from build123d import *

# Parameters (mm, degrees)
EXTRUDE_START   = -375
EXTRUDE_1_DEPTH = 750


with BuildPart() as part:
    # Extrude sketch 1 → Extrude 1 (new body)
    with BuildSketch(Plane(origin=(0, 0, 0), x_dir=(1, 0, 0), z_dir=(0, 1, 0)).offset(EXTRUDE_START)):
        with BuildLine():
            Line((20, 16), (20, -16))
            ThreePointArc((20, -16), (18.828427125, -18.828427125), (16, -20))
            Line((16, -20), (-16, -20))
            ThreePointArc((-16, -20), (-18.828427125, -18.828427125), (-20, -16))
            Line((-20, -16), (-20, 16))
            ThreePointArc((-20, 16), (-18.828427125, 18.828427125), (-16, 20))
            Line((-16, 20), (16, 20))
            ThreePointArc((16, 20), (18.828427125, 18.828427125), (20, 16))
        make_face()
        with BuildLine():
            Line((17, 15.5), (17, -15.5))
            ThreePointArc((17, -15.5), (16.560660172, -16.560660172), (15.5, -17))
            Line((15.5, -17), (-15.5, -17))
            ThreePointArc((-15.5, -17), (-16.560660172, -16.560660172), (-17, -15.5))
            Line((-17, -15.5), (-17, 15.5))
            ThreePointArc((-17, 15.5), (-16.560660172, 16.560660172), (-15.5, 17))
            Line((-15.5, 17), (15.5, 17))
            ThreePointArc((15.5, 17), (16.560660172, 16.560660172), (17, 15.5))
        make_face(mode=Mode.SUBTRACT)
    extrude(amount=EXTRUDE_1_DEPTH)


solid = part.part
Here's how the part is built. I have some questions about the finished solid (model axes, mm). A direction names the side the tool comes from. Coordinates: 2 decimals unless noted, no trailing zeros. Loops run counter-clockwise (first coordinate to the right, second up) from the corner with the lowest first, then second, coordinate; pieces in that order, holes last. Notation, with made-up numbers: (-37.5, -28) -> (8.5, -28) arc R23 cw to (8.5, 9) -> close; hole circle Ø6 at (75, -18). An arc over 180 degrees is marked (long way). Use one line per item in the form item = value. Start each with the question number.
(1) If we section it at C-C (z = 9): Please give me the cut outline in (x, y).
(2) Will this pin go through, and if not, where does the flat tip stop? pin 1 (8 mm diameter, centred on x = 8.5, z = 9.5, fed in from -Y).
(3) We'd pull the mould along X, two halves only. Please class faces 1 (the face through (20, -5, 0)), 2 (the face through (18, -375, 0)), 3 (the face through (0, -5, 17)): pulls with the +X half, pulls with the -X half, needs draft (parallel to the pull), parting line crosses it, or undercut.
(4) On a 3-axis mill with a long thin cutter (end or side, diameter ignored), from which of +Z, -Z, +X, -X, +Y, -Y can I reach the whole of each face in a straight line? I mean faces 4 (the face through (0, -5, -17)), 5 (the face through (0, -5, -20)). Say none if no direction works.
(5) Please list where these lines run through material, in increasing order: line 1 along Z through (x, y) = (11, 138); line 2 along X through (y, z) = (-20.5, -16).
(6) If we section it at B-B (y = 327.5): Please give me the cut outline in (x, z).
(7) If we section it at A-A (x = 7): Please give me the cut outline in (y, z).
Verdict:
q1.outline = (-20, -375) -> (-17, -375) -> (-17, 375) -> (-20, 375) -> close; (17, -375) -> (20, -375) -> (20, 375) -> (17, 375) -> close
q2.pin_1 = through
q3.face_1 = pulls with the +X half
q3.face_2 = needs draft
q3.face_3 = undercut
q4.face_4 = +Y, -Y
q4.face_5 = -Z, +X, -X, +Y, -Y
q5.line_1 = -20 to -17, 17 to 20
q5.line_2 = -20 to -16.91, 16.91 to 20
q6.outline = (-20, -16) arc R4 ccw to (-16, -20) -> (16, -20) arc R4 ccw to (20, -16) -> (20, 16) arc R4 ccw to (16, 20) -> (-16, 20) arc R4 ccw to (-20, 16) -> close; hole (-17, -15.5) arc R1.5 ccw to (-15.5, -17) -> (15.5, -17) arc R1.5 ccw to (17, -15.5) -> (17, 15.5) arc R1.5 ccw to (15.5, 17) -> (-15.5, 17) arc R1.5 ccw to (-17, 15.5) -> close
q7.outline = (-375, -20) -> (375, -20) -> (375, -17) -> (-375, -17) -> close; (-375, 17) -> (375, 17) -> (375, 20) -> (-375, 20) -> close
